from build123d import *

# Parameters (mm, degrees)
SKETCH1_W           = 80
SKETCH1_H           = 40
BOSS_EXTRUDE1_DEPTH = 10
SKETCH2_W           = 40
SKETCH2_H           = 40
BOSS_EXTRUDE2_DEPTH = 10
SKETCH3_R           = 5
CUT_EXTRUDE1_DEPTH  = 10
SKETCH4_R           = 5
BOSS_EXTRUDE3_DEPTH = 10
SKETCH5_R           = 5
CUT_EXTRUDE2_DEPTH  = 10


with BuildPart() as part:
    # Sketch1 → Boss-Extrude1 (new body)
    with BuildSketch(Plane(origin=(0, 0, 0), x_dir=(1, 0, 0), z_dir=(0, 1, 0))):
        Rectangle(SKETCH1_W, SKETCH1_H)
    extrude(amount=BOSS_EXTRUDE1_DEPTH)

    # Sketch2 → Boss-Extrude2 (add)
    with BuildSketch(Plane(origin=(0, 10, 0), x_dir=(1, 0, 0), z_dir=(0, 1, 0))):
        Rectangle(SKETCH2_W, SKETCH2_H)
    extrude(amount=BOSS_EXTRUDE2_DEPTH)

    # Sketch3 → Cut-Extrude1 (cut)
    with BuildSketch(Plane(origin=(0, 20, 0), x_dir=(1, 0, 0), z_dir=(0, 1, 0))):
        Circle(SKETCH3_R)
    extrude(amount=-CUT_EXTRUDE1_DEPTH, mode=Mode.SUBTRACT)

    # Sketch4 → Boss-Extrude3 (add)
    with BuildSketch(Plane(origin=(0, 10, 0), x_dir=(1, 0, 0), z_dir=(0, 1, 0))):
        Circle(SKETCH4_R)
    extrude(amount=BOSS_EXTRUDE3_DEPTH)

    # Sketch5 → Cut-Extrude2 (cut)
    with BuildSketch(Plane(origin=(0, 20, 0), x_dir=(1, 0, 0), z_dir=(0, 1, 0))):
        Circle(SKETCH5_R)
    extrude(amount=-CUT_EXTRUDE2_DEPTH, mode=Mode.SUBTRACT)


solid = part.part
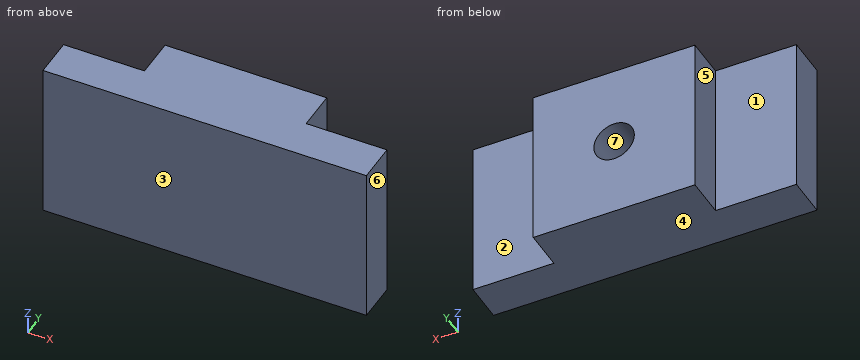
For this review, take the finished solid that the model builds, in its own axes (mm). Face numbers are marked on the shaded views. A direction names the side the tool comes from. Round coordinates to 2 decimals unless told otherwise and drop trailing zeros. Loops run counter-clockwise (first coordinate to the right, second up) from the corner with the lowest first, then second, coordinate; pieces in that order, holes last. Notation, with made-up numbers: (-14, -38) - (34, -38) arc R23 cw to (34, -29) - close; hole circle Ø2 at (12.25, -9.5). An arc over 180 degrees is marked (long way). Answer as CSV lines item,"result".
(1) Consider section B-B on x = 0. Give the boundary of the cut face in (y, z).
Checked values:
outline,"(0, -20) - (20, -20) - (20, -5) - (10, -5) - (10, 5) - (20, 5) - (20, 20) - (0, 20) - close"
(2) Consider section C-C on z = 0. Give the boundary of the cut face in (x, y).
Checked values:
outline,"(-40, 0) - (40, 0) - (40, 10) - (20, 10) - (20, 20) - (5, 20) - (5, 10) - (-5, 10) - (-5, 20) - (-20, 20) - (-20, 10) - (-40, 10) - close"
(3) Consider section D-D on x = -34. Give the boundary of the cut face in (y, z), then the cut area to 3 significant figures.
Checked values:
outline,"(0, -20) - (10, -20) - (10, 20) - (0, 20) - close"
area,"400 mm2"
(4) Insertion check: P1, Ø3, axis at y = 14.5, z = -1, coming from the +X side; P2, Ø10, axis at x = -13.5, z = -5.5, coming from the -Y side; P3, Ø10, axis at x = -32.5, z = -6.5, coming from the +Y side. Each pin has a flat end and moves straight along its axis. Give the tip position at first contact, or say it passes through.
Checked values:
P1,"stops at x = 20"
P2,"stops at y = 0"
P3,"stops at y = 10"
(5) Wall thickness on line 1 (Z direction, x = 0, y = 12.5); line 2 (Y direction, x = 31.5, z = -12): over which ranges is each line inside the solid? List them lowest first.
Checked values:
line 1,"z = -20 to -5, 5 to 20"
line 2,"y = 0 to 10"
(6) Tool access review of the marked faces 1, 2 and 3: name each direction out of +Z, -Z, +X, -X, +Y, -Y from which nothing blocks a thin tool from reaching the whole face with its end or side.
Checked values:
face 1,"+Z, -Z, -X, +Y"
face 2,"+Z, -Z, +X, +Y"
face 3,"+Z, -Z, +X, -X, -Y"
(7) Mouldability with a two-part tool opening along X and no side actions: class the marked faces 4, 5, 6 and 7 as +X half, -X half, draft (parallel to the pull), parting line (faces both ways), or undercut.
Checked values:
face 4,"draft"
face 5,"-X half"
face 6,"+X half"
face 7,"undercut"
(8) Consider section A-A on z = 14.5. Give the boundary of the cut face in (x, y).
Checked values:
outline,"(-40, 0) - (40, 0) - (40, 10) - (20, 10) - (20, 20) - (-20, 20) - (-20, 10) - (-40, 10) - close"
